Input: part model. Units: mm. Frame: model coordinates. A direction names the side the tool comes from. Round coordinates to 2 decimals unless told otherwise and drop trailing zeros. Loops run counter-clockwise (first coordinate to the right, second up) from the corner with the lowest first, then second, coordinate; pieces in that order, holes last. Notation, with made-up numbers: (-7.75, 76.25) - (35.25, 76.25) arc R19 ccw to (35.25, 111.25) - close; hole circle Ø1 at (-21, 43). An arc over 180 degrees is marked (long way). Use CSV: the item, a comma, the result in double quotes. Start each with the question number.
1. Pin query (flat end, axial travel): P1, Ø8, axis at x = -18, z = 22, coming from the +Y side; P2, Ø6, axis at x = 22, z = 8, coming from the -Y side; P3, Ø4.5, axis at x = -44, z = 11, coming from the +Y side. Return the tip coordinate at first contact, or that it passes through.
2. Cut plane C-C (x = 0). Return loops of the section in (y, z), and give its area (3 significant figures).
3. Cut plane D-D (y = -31). Return loops of the section in (x, z).
4. Cut plane B-B (z = 15.25). Return loops of the section in (x, y).
5. Material intervals for probe 1 along X at (y, z) = (-35.8, 7); probe 2 along X at (y, z) = (1, 25.25); probe 3 along Z at (x, y) = (45, -36), sorted ascending. Write a range as from..to.
6. Cut plane A-A (y = -18). Return loops of the section in (x, z), and give its area (3 significant figures).
7. Pull-direction query (X, two-part tool) for faces 5 (the cylindrical face through (42.838, -36.594, 22.059)), 6 (the flat face through (39, -37.9, 14)), 7 (the flat face through (-52.9, -36, 14)), 8 (the flat face through (-26.45, -36, 14)); classes: +X half, -X half, draft (parallel to the pull), parting line (faces both ways), or undercut.
8. Access query for faces 1 (the flat face through (32, -14, 28)), 2 (the flat face through (-28.614, -23.641, 13.804)), 3 (the flat face through (-45, -33.7, 14)), 4 (the flat face through (26.45, -36, 14)). Directions: +Z, -Z, +X, -X, +Y, -Y. A direction counts if a zero-diameter tool reaches every point of the face in a straight line with its end or side. Return the directions, or none.
```python
from build123d import *

# Parameters (mm, degrees)
PAD_DEPTH        = 28
HOLE_D           = 3
HOLE_DEPTH       = 25
HOLE_CSINK_D     = 6.1
HOLE_CSINK_ANGLE = 90


with BuildPart() as part:
    # Sketch → Pad (new body)
    with BuildSketch(Plane.XY):
        with BuildLine():
            ThreePointArc((30.717917, -13.86), (0, 33.7), (-30.717917, -13.86))
            Line((-30.717917, -13.86), (-26.45, -33.7))
            Line((-26.45, -33.7), (-26.45, -37.9))
            Line((-52.9, -37.9), (-26.45, -37.9))
            Line((-52.9, -33.7), (-52.9, -37.9))
            Line((-37.9, -33.7), (-52.9, -33.7))
            Line((-37.9, 0), (-37.9, -33.7))
            ThreePointArc((37.9, 0), (0, 37.9), (-37.9, 0))
            Line((37.9, 0), (37.9, -33.7))
            Line((52.9, -33.7), (37.9, -33.7))
            Line((52.9, -37.9), (52.9, -33.7))
            Line((26.45, -37.9), (52.9, -37.9))
            Line((26.45, -33.7), (26.45, -37.9))
            Line((30.717917, -13.86), (26.45, -33.7))
        make_face()
    extrude(amount=PAD_DEPTH)

    # Hole
    with Locations(Plane(origin=(0, -33.7, 0), x_dir=(-1, 0, 0), z_dir=(0, 1, 0))):
        with Locations((45.4, 7), (-45.4, 7), (-44.336327, 21.992761), (44.318888, 22.009038)):
            CounterSinkHole(HOLE_D / 2, HOLE_CSINK_D / 2, depth=HOLE_DEPTH, counter_sink_angle=HOLE_CSINK_ANGLE)


solid = part.part
```
Established:
1,P1,"stops at y = 35.22"
1,P2,"stops at y = 22.6"
1,P3,"stops at y = -33.7"
2,outline,"(33.7, 0) - (37.9, 0) - (37.9, 28) - (33.7, 28) - close"
2,area,"118 mm2"
3,outline,"(-37.9, 0) - (-27.03, 0) - (-27.03, 28) - (-37.9, 28) - close; (27.03, 0) - (37.9, 0) - (37.9, 28) - (27.03, 28) - close"
4,outline,"(-52.9, -37.9) - (-26.45, -37.9) - (-26.45, -33.7) - (-30.72, -13.86) arc R33.7 cw (long way) to (30.72, -13.86) - (26.45, -33.7) - (26.45, -37.9) - (52.9, -37.9) - (52.9, -33.7) - (37.9, -33.7) - (37.9, 0) arc R37.9 ccw to (-37.9, 0) - (-37.9, -33.7) - (-52.9, -33.7) - close"
5,probe 1,"x = -52.9..-46.9, -43.9..-26.45, 26.45..43.9, 46.9..52.9"
5,probe 2,"x = -37.89..-33.69, 33.69..37.89"
5,probe 3,"z = 0..5.55, 8.45..20.65, 23.34..28"
6,outline,"(-37.9, 0) - (-29.83, 0) - (-29.83, 28) - (-37.9, 28) - close; (29.83, 0) - (37.9, 0) - (37.9, 28) - (29.83, 28) - close"
6,area,"452 mm2"
7,face 5,"undercut"
7,face 6,"draft"
7,face 7,"-X half"
7,face 8,"undercut"
8,face 1,"+Z, +X, -X, +Y, -Y"
8,face 2,"+Z, -Z"
8,face 3,"+Z, -Z, -X, +Y"
8,face 4,"+Z, -Z, -Y"
